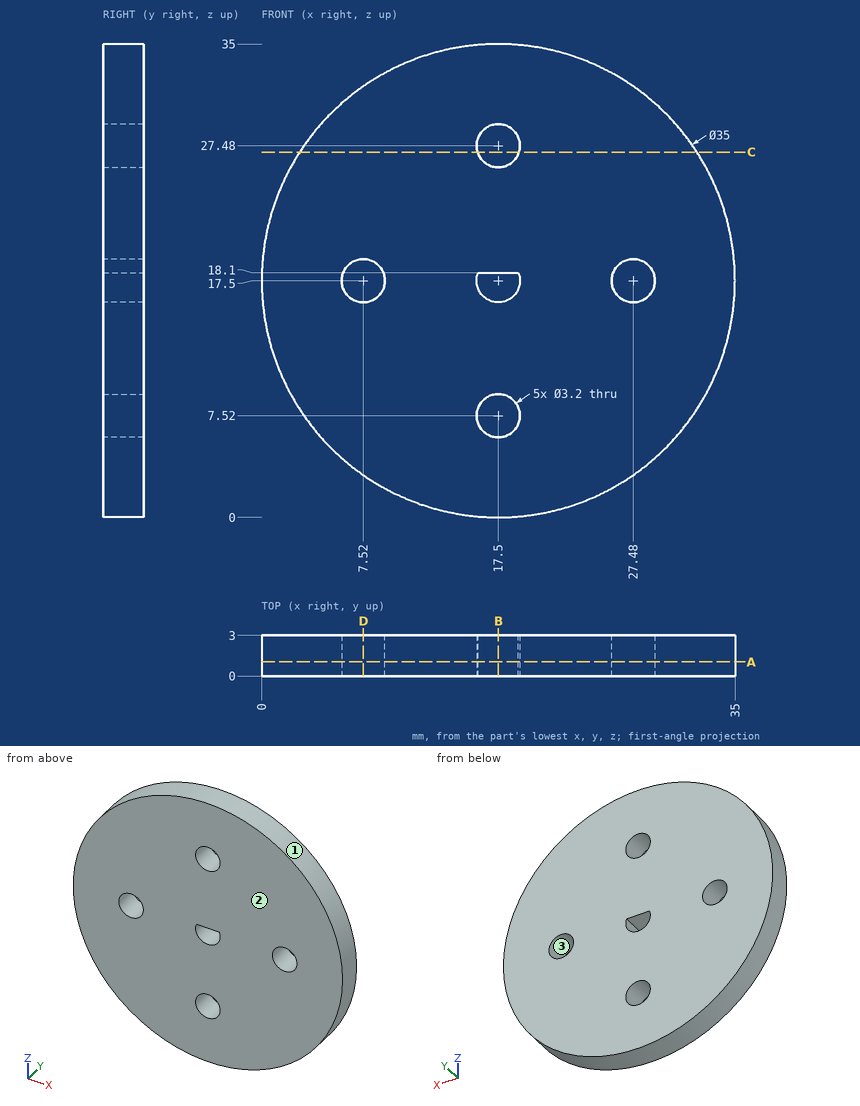
Drawing for the job (mm, zero at the part's lowest x, y, z). Give positions to 0.01 mm unless a question says otherwise; leave off trailing zeros. Order: outer loops, then holes, each group sorted by start corner. A loop starts at its lowest first (then second) coordinate and runs counter-clockwise, first axis right, second up. Notation, with made-up numbers: M 25.5,25.25 L 37.5,25.25 A24 cw 37.5,44.25 Z; hole C 45,0 d6. An arc over 180 degrees is marked long. Put each result on its own line as item: value. Start each with the question number.
(1) Mould opens along X. For the marked faces 1, 2 and 3 say: +X half, -X half, draft (parallel to the pull), parting line (faces both ways), or undercut.
(2) Saw through at B-B, the plane x = 17.5. Write the cut outline in (y, z), then the cut area to 3 significant figures.
(3) Drill centre lines: line 1 along Z through (x, y) = (17.5, 1.4); line 2 along Z through (x, y) = (7.52, 1.7). Where is each one in solid material? Low to high.
(4) Saw through at D-D, the plane x = 7.52. Write the cut outline in (y, z), then the cut area to 4 significant figures.
(5) Flat gauge pins, fed straight in: pin 1 Ø1 at (y, z) = (1.5, 11.5) entering from -X; pin 2 Ø1 at (x, y) = (9, 1) entering from +Z. Where does each tip first touch, or does it go through?
(6) Saw through at C-C, the plane z = 27. Write the cut outline in (x, y).
(7) Saw through at A-A, the plane y = 1.05. Write the cut outline in (x, z), then the cut area to 3 significant figures.
Check result:
1. face 1: parting line
1. face 2: draft
1. face 3: undercut
2. outline: M 0,0 L 3,0 L 3,5.92 L 0,5.92 Z; M 0,9.12 L 3,9.12 L 3,15.9 L 0,15.9 Z; M 0,18.1 L 3,18.1 L 3,25.88 L 0,25.88 Z; M 0,29.08 L 3,29.08 L 3,35 L 0,35 Z
2. area: 79.2 mm2
3. line 1: z = 0 to 5.92, 9.12 to 15.9, 18.1 to 25.88, 29.08 to 35
3. line 2: z = 3.12 to 15.9, 19.1 to 31.88
4. outline: M 0,3.12 L 3,3.12 L 3,15.9 L 0,15.9 Z; M 0,19.1 L 3,19.1 L 3,31.88 L 0,31.88 Z
4. area: 76.65 mm2
5. pin 1: stops at x = 0.89
5. pin 2: stops at z = 33.06
6. outline: M 2.8,0 L 15.97,0 L 15.97,3 L 2.8,3 Z; M 19.03,0 L 32.2,0 L 32.2,3 L 19.03,3 Z
7. outline: C 17.5,17.5 d35; hole C 7.52,17.5 d3.2; hole C 17.5,7.52 d3.2; hole C 17.5,27.48 d3.2; hole M 16.02,18.1 A1.6 ccw long 18.98,18.1 Z; hole C 27.48,17.5 d3.2
7. area: 924 mm2
